Check sheet for the modelled part. Datum: model origin and axes. Units: mm. Coordinates: 2 decimals unless noted, no trailing zeros. Loops run counter-clockwise (first coordinate to the right, second up) from the corner with the lowest first, then second, coordinate; pieces in that order, holes last. Notation, with made-up numbers: (74, 43.5) -> (117, 43.5) arc R11 ccw to (117, 61.5) -> close; hole circle Ø8 at (32, 82). An arc over 180 degrees is marked (long way). Use CSV: the item, a comma, the result in double quotes. Start each with the question number.
1. Sectioned sample at A-A, the plane x = 106.5. Record the cut outline in (y, z), and give its area (3 significant figures).
2. Release check for a two-part mould opening along X. For faces 1 (the face through (102.83, 1.52, -25.24)), 2 (the face through (-2, 0, -2)) record: pulls with the +X half, pulls with the -X half, needs draft (parallel to the pull), parting line crosses it, or undercut.
3. Thickness scan on L1, parallel to X at y = 1.15, z = -35; L2, parallel to X at y = 1.4, z = 40; L3, parallel to Z at x = -125, y = 1.3. Record the ranges inside material, lowest first.
```python
from build123d import *

# Parameters (mm, degrees)
SKETCH1_W           = 350.000000098
SKETCH1_H           = 350.000000098
SKETCH1_R           = 1.6
BOSS_EXTRUDE1_DEPTH = 3
SKETCH2_R           = 10
SKETCH2_R_2         = 1.6
CUT_EXTRUDE1_DEPTH  = 3


with BuildPart() as part:
    # Sketch1 → Boss-Extrude1 (new body)
    with BuildSketch(Plane(origin=(0, 0, 0), x_dir=(1, 0, 0), z_dir=(0, 1, 0))):
        Rectangle(SKETCH1_W, SKETCH1_H)
        with Locations((-150, 150)):
            Circle(SKETCH1_R, mode=Mode.SUBTRACT)
        with Locations((-150, -150)):
            Circle(SKETCH1_R, mode=Mode.SUBTRACT)
        with Locations((150, -150)):
            Circle(SKETCH1_R, mode=Mode.SUBTRACT)
        with Locations((150, 150)):
            Circle(SKETCH1_R, mode=Mode.SUBTRACT)
    extrude(amount=BOSS_EXTRUDE1_DEPTH)

    # Sketch2 → Cut-Extrude1 (cut)
    with BuildSketch(Plane(origin=(0, 3, 0), x_dir=(1, 0, 0), z_dir=(0, 1, 0))):
        with Locations((-105, 35)):
            Circle(SKETCH2_R)
        with Locations((105, 35)):
            Circle(SKETCH2_R)
        with Locations((-20.861599962, 154.028549732)):
            Circle(SKETCH2_R_2)
        with Locations((-24.234411868, 87.928549732)):
            Circle(SKETCH2_R_2)
        with Locations((21.048400038, 154.028549732)):
            Circle(SKETCH2_R_2)
        with Locations((24.155588132, 87.928549732)):
            Circle(SKETCH2_R_2)
        with Locations((-125, 0)):
            Circle(SKETCH2_R_2)
        with Locations((-85, 0)):
            Circle(SKETCH2_R_2)
        with Locations((-125, -40)):
            Circle(SKETCH2_R_2)
        with Locations((-85, -40)):
            Circle(SKETCH2_R_2)
        with Locations((85, 0)):
            Circle(SKETCH2_R_2)
        with Locations((125, 0)):
            Circle(SKETCH2_R_2)
        with Locations((85, -40)):
            Circle(SKETCH2_R_2)
        with Locations((125, -40)):
            Circle(SKETCH2_R_2)
    extrude(amount=-CUT_EXTRUDE1_DEPTH, mode=Mode.SUBTRACT)


solid = part.part
```
Completed:
1,outline,"(0, -175) -> (3, -175) -> (3, -44.89) -> (0, -44.89) -> close; (0, -25.11) -> (3, -25.11) -> (3, 175) -> (0, 175) -> close"
1,area,"991 mm²"
2,face 1,"undercut"
2,face 2,"needs draft"
3,L1,"-175 to -115, -95 to 95, 115 to 175"
3,L2,"-175 to -126.6, -123.4 to -86.6, -83.4 to 83.4, 86.6 to 123.4, 126.6 to 175"
3,L3,"-175 to -1.6, 1.6 to 38.4, 41.6 to 175"
